Autodesk Inventor part; units mm, degrees
ref_plane "YZ Plane" through (0, 0, 0) normal (1, 0, 0) x (0, 1, 0)
ref_plane "XZ Plane" through (0, 0, 0) normal (0, 1, 0) x (-1, 0, 0)
ref_plane "XY Plane" through (0, 0, 0) normal (0, 0, 1) x (1, 0, 0)
sketch "Sketch1" plane through (0, 0, 0) normal (0, 0, 1) x (1, 0, 0)
  circle A0 centre (0, 0) radius 1.5
  circle A1 centre (0, 0) radius 2.25
  dimension "d0" = 3
  dimension "d2" = 4.5
extrude "Extrusion1" add sketch "Sketch1" along normal blind 3
sketch "Sketch3" plane through (0, 0, 0) normal (0, 0, 1) x (1, 0, 0)
  circle A0 centre (0, 0) radius 2.25
  circle A1 centre (0, 0) radius 2.75
  dimension "d10" = 4.5
  dimension "d11" = 5.5
extrude "Extrusion3" add sketch "Sketch3" along normal blind 2.5
sketch "Sketch4" plane through (0, 0, 0) normal (0, 0, -1) x (-1, 0, 0)
  circle A0 centre (0, 0) radius 2.25
  circle A1 centre (0, 0) radius 2.75
  dimension "d14" = 4.5
  dimension "d15" = 5.5
extrude "Extrusion4" cut sketch "Sketch4" against normal blind 0.5
sketch "Sketch5" plane through (0, 0, 0) normal (0, 0, 1) x (1, 0, 0)
  circle A0 centre (0, 0) radius 2.75
  circle A1 centre (0, 0) radius 3.5
  dimension "d18" = 5.5
  dimension "d19" = 7
extrude "Extrusion5" add sketch "Sketch5" along normal blind 3
properties part number "2P.03.01.00.01.IM.Bearing373" material "Aluminum 6061"
The listing builds one solid part. Answer for the finished solid, in the listing's coordinates (mm). A direction names the side the tool comes from. Coordinates: 2 decimals unless noted, no trailing zeros. Order: outer loops, then holes, each group sorted by start corner. A loop starts at its lowest first (then second) coordinate and runs counter-clockwise, first axis right, second up. Notation, with made-up numbers: (-2.5, -16.75) -> (27.5, -16.75) arc R26 ccw to (27.5, 4.25) -> close; hole circle Ø9 at (13.25, 76). An arc over 180 degrees is marked (long way). Answer in a Markdown table with one row per item. Add a question column.
Item 1: This flat-tipped pin is pushed along its axis until it touches: P1, Ø1, axis at x = 2.5, z = 2, coming from the +Y side. Where does it stop, or does it pass through?
Item 2: Which of the six approach directions +Z, -Z, +X, -X, +Y, -Y give full straight-line access (tool end or side, diameter ignored) to faces 5 (the face through (-2, 0, 3)), 6 (the face through (-0.596, 2.685, 0.246)), 7 (the face through (-0.29, -2.23, 2.75))?
Item 3: Determine the mould class of faces 1 (the face through (-0.596, 2.685, 2.746)), 2 (the face through (-1.5, -0.07, 1.48)), 3 (the face through (3.233, 1.341, 1.479)), 4 (the face through (-3, -1, 0)) for opening direction X: +X half, -X half, draft (parallel to the pull), parting line (faces both ways), or undercut.
Item 4: Find section A-A (x = 0). Write down the section's boundary in (y, z), then the cut area to 3 significant figures.
Item 5: Find the intervals of material crossed by L1, parallel to Y at x = 0, z = 2.75; L2, parallel to Y at x = 0, z = 2.3; L3, parallel to Y at x = -0.75, z = 2.6, in increasing order. Write a range as from..to.
Item 6: Find section C-C (z = 2.7). Write down the section's boundary in (x, y).
Item 7: Find section D-D (y = 1.75). Write down the section's boundary in (x, z).
Result set:
| question | item | result |
|---|---|---|
| 1 | P1 | stops at y = 2.87 |
| 2 | face 5 | +Z, +X, -X, +Y, -Y |
| 2 | face 6 | -Z |
| 2 | face 7 | +Z |
| 3 | face 1 | undercut |
| 3 | face 2 | undercut |
| 3 | face 3 | parting line |
| 3 | face 4 | draft |
| 4 | outline | (-3.5, 0) -> (-2.75, 0) -> (-2.75, 0.5) -> (-2.25, 0.5) -> (-2.25, 0) -> (-1.5, 0) -> (-1.5, 3) -> (-2.25, 3) -> (-2.25, 2.5) -> (-2.75, 2.5) -> (-2.75, 3) -> (-3.5, 3) -> close; (1.5, 0) -> (2.25, 0) -> (2.25, 0.5) -> (2.75, 0.5) -> (2.75, 0) -> (3.5, 0) -> (3.5, 3) -> (2.75, 3) -> (2.75, 2.5) -> (2.25, 2.5) -> (2.25, 3) -> (1.5, 3) -> close |
| 4 | area | 11.0 mm² |
| 5 | L1 | y = -3.5..-2.75, -2.25..-1.5, 1.5..2.25, 2.75..3.5 |
| 5 | L2 | y = -3.5..-1.5, 1.5..3.5 |
| 5 | L3 | y = -3.42..-2.65, -2.12..-1.3, 1.3..2.12, 2.65..3.42 |
| 6 | outline | circle Ø7 at (0, 0); circle Ø4.5 at (0, 0); hole circle Ø5.5 at (0, 0); hole circle Ø3 at (0, 0) |
| 7 | outline | (-3.03, 0) -> (-2.12, 0) -> (-2.12, 0.5) -> (-1.41, 0.5) -> (-1.41, 0) -> (1.41, 0) -> (1.41, 0.5) -> (2.12, 0.5) -> (2.12, 0) -> (3.03, 0) -> (3.03, 3) -> (2.12, 3) -> (2.12, 2.5) -> (1.41, 2.5) -> (1.41, 3) -> (-1.41, 3) -> (-1.41, 2.5) -> (-2.12, 2.5) -> (-2.12, 3) -> (-3.03, 3) -> close |
